The model under review builds one solid part; all positions refer to its coordinate system, in mm. Face numbers are marked on the shaded views. A direction names the side the tool comes from. Coordinates: 2 decimals unless noted, no trailing zeros. Write each loop counter-clockwise with the first axis right and the second up, starting at its lowest first coordinate (ties: lowest second). Pieces come first, ordered by that corner, then holes. Notation, with made-up numbers: M -35,52.5 L -22,52.5 A11 cw -22,59.5 Z; hole C 18.5,47.25 d10. An arc over 180 degrees is marked long. Answer as CSV lines item,"result". Start each with the question number.
Autodesk Inventor part; units mm, degrees
ref_plane "YZ Plane" through (0, 0, 0) normal (1, 0, 0) x (0, 1, 0)
ref_plane "XZ Plane" through (0, 0, 0) normal (0, 1, 0) x (-1, 0, 0)
ref_plane "XY Plane" through (0, 0, 0) normal (0, 0, 1) x (1, 0, 0)
sketch "Sketch1" plane through (0, 0, 0) normal (0, 0, 1) x (1, 0, 0)
  line L0 (0, 0) -> (15, 0)
  line L1 (15, 0) -> (15, -15)
  line L2 (15, -15) -> (45, -15)
  line L3 (45, -15) -> (45, 75)
  line L4 (45, 75) -> (15, 75)
  line L5 (15, 75) -> (15, 47)
  line L6 (15, 47) -> (0, 47)
  line L7 (0, 0) -> (0, 47) construction
  line L8 (0, 0) -> (-15, 0)
  line L9 (-15, 0) -> (-15, -15)
  line L10 (-15, -15) -> (-45, -15)
  line L11 (-45, -15) -> (-45, 75)
  line L12 (-45, 75) -> (-15, 75)
  line L13 (-15, 75) -> (-15, 47)
  line L14 (-15, 47) -> (0, 47)
  dimension "d0" = 47
  dimension "d1" = 28
  dimension "d2" = 30
  dimension "d3" = 15
  dimension "d4" = 90
extrude "Extrusion1" add sketch "Sketch1" along normal blind 90
sketch "Sketch2" plane through (-45, -15, 0) normal (-1, 0, 0) x (0, 0, 1)
  line L0 (0, 90) -> (0, 0)
  line L1 (0, 0) -> (90, 0)
  line L2 (90, 90) -> (90, 0)
  line L3 (0, 90) -> (90, 90)
  line L4 (90, 15) -> (90, 0)
  line L5 (90, 0) -> (52.5, 90)
  line L6 (0, 90) -> (90, 90)
  line L7 (37.5, 90) -> (0, 0)
  line L8 (30, 0) -> (30, 15)
  line L9 (30, 15) -> (60, 15)
  line L10 (60, 15) -> (60, 0)
  point P0 (0, 15)
  point P1 (45, 15)
  point P2 (45, 0)
  dimension "d12" = 30
  dimension "d13" = 15
extrude "Extrusion2" cut sketch "Sketch2" against normal blind 90 contours L3 L7 L0 | L8 L9 L10 L1 | L3 L2 L5
properties part number "b4"
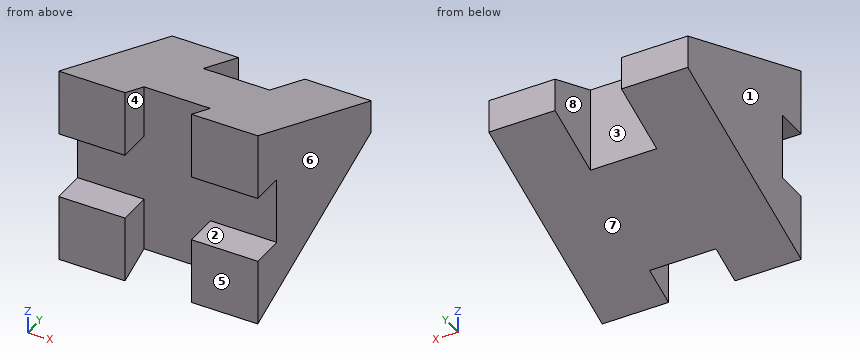
1) Take a section at D-D on x = -30. Give the boundary of the cut face in (y, z), and give its area (4 significant figures).
2) Take a section at A-A on y = 57. Give the boundary of the cut face in (x, z), and give its area (3 significant figures).
3) Take a section at B-B on z = 77.5. Give the boundary of the cut face in (x, y), and give its area (3 significant figures).
4) Tool access review of the marked faces 1, 2, 3, 4 and 5: name each direction out of +Z, -Z, +X, -X, +Y, -Y from which nothing blocks a thin tool from reaching the whole face with its end or side.
5) Take a section at C-C on y = -4.5. Give the boundary of the cut face in (x, z) (3 decimals), and give its area (4 significant figures).
6) Mouldability with a two-part tool opening along X and no side actions: class the marked faces 6, 7 and 8 as +X half, -X half, draft (parallel to the pull), parting line (faces both ways), or undercut.
7) Clearance check with flat-ended pins moving along their axes: pin 1 Ø15 at (x, z) = (-7, 42.5) entering from +Y; pin 2 Ø3 at (x, z) = (-31, 38.5) entering from -Y; pin 3 Ø4.5 at (x, y) = (-29.5, -9.5) entering from +Z. State where each tip first meets the part, or that it passes through.
8) To check wall thickness, follow line 1 (X direction, y = 67, z = 53.5); line 2 (Y direction, x = 3.5, z = 40.5); line 3 (Y direction, x = 18.5, z = 42). State the ranges of each line that lie inside material, in increasing order. Write a range as [from, to].
Results:
1,outline,"M -15,0 L 75,37.5 L 75,52.5 L -15,90 L -15,60 L 0,60 L 0,30 L -15,30 Z"
1,area,"4,275 mm²"
2,outline,"M -45,30 L -15,30 L -15,60 L -45,60 Z; M 15,30 L 45,30 L 45,60 L 15,60 Z"
2,area,"1,800 mm²"
3,outline,"M -45,-15 L -15,-15 L -15,0 L 15,0 L 15,-15 L 45,-15 L 45,15 L -45,15 Z"
3,area,"2,250 mm²"
4,face 1,"+Z, -Z, -X, +Y, -Y"
4,face 2,"+X, -X, -Y"
4,face 3,"+Z, -Z, +Y"
4,face 4,"+Z, -Z, -Y"
4,face 5,"+Z, -Z, +X, -X, -Y"
5,outline,"M -45,4.375 L -15,4.375 L -15,30 L -45,30 Z; M -45,60 L -15,60 L -15,85.625 L -45,85.625 Z; M 15,4.375 L 45,4.375 L 45,30 L 15,30 Z; M 15,60 L 45,60 L 45,85.625 L 15,85.625 Z"
5,area,"3,075 mm²"
6,face 6,"+X half"
6,face 7,"draft"
6,face 8,"undercut"
7,pin 1,"stops at y = 47"
7,pin 2,"stops at y = 0"
7,pin 3,"stops at z = 88.65"
8,line 1,"x = [-45, -15], [15, 45]"
8,line 2,"y = [0, 47]"
8,line 3,"y = [0, 75]"
